Read the model definition and answer for the solid it produces. Units are mm, in the model's axes. Face numbers are marked on the shaded views. A direction names the side the tool comes from. Give positions to 0.01 mm unless a question says otherwise; leave off trailing zeros. Write each loop counter-clockwise with the first axis right and the second up, starting at its lowest first coordinate (ties: lowest second). Pieces come first, ordered by that corner, then holes. Notation, with made-up numbers: (3, -14.75) -> (35, -14.75) arc R8 cw to (35, -0.75) -> close; hole circle Ø4 at (66.25, 28.25). An arc over 180 degrees is marked (long way). Put each result on its own line as item: value. Start each with the question number.
Autodesk Inventor part; units mm, degrees
ref_plane "YZ Plane" through (0, 0, 0) normal (1, 0, 0) x (0, 1, 0)
ref_plane "XZ Plane" through (0, 0, 0) normal (0, 1, 0) x (-1, 0, 0)
ref_plane "XY Plane" through (0, 0, 0) normal (0, 0, 1) x (1, 0, 0)
sketch "Sketch1" plane through (0, 0, 0) normal (1, 0, 0) x (0, 1, 0)
  line L0 (0, 0) -> (20, 0)
  line L1 (20, 0) -> (20, -17)
  line L2 (20, -17) -> (0, -17)
  line L3 (0, -17) -> (0, 0)
  dimension "d0" = 20
  dimension "d1" = 17
extrude "Extrusion1" add sketch "Sketch1" along normal blind 3
sketch "Sketch2" plane through (0, 0, -17) normal (0, -1, 0) x (1, 0, 0)
  line L0 (3, 0) -> (3, 17)
  line L1 (3, 17) -> (-17, 17)
  line L2 (-17, 17) -> (-17, 0)
  line L3 (-17, 0) -> (3, 0)
  line L4 (3, 0) -> (3, 17)
  line L5 (-17, 17) -> (-17, 0)
  line L6 (0, 0) -> (-17, 0)
  line L7 (0, 17) -> (0, 0)
  line L8 (-17, 17) -> (0, 17)
  line L9 (-10, 8.5) -> (-7, 8.5) construction
  line L10 (-10, 5) -> (-7, 5)
  line L11 (-7, 12) -> (-10, 12)
  arc A0 (-10, 12) -> (-10, 5) centre (-10, 8.5) ccw
  arc A1 (-7, 5) -> (-7, 12) centre (-7, 8.5) ccw
  point P0 (0, 17)
  point P1 (0, 0)
  point P2 (-8.5, 8.5)
  dimension "d4" = 20
  dimension "d15" = 7
  dimension "d16" = 3
  dimension "d17" = 7
  dimension "d18" = 17
  dimension "d19" = 17
  dimension "d20" = 8.5
extrude "Extrusion2" add sketch "Sketch2" against normal blind 3 contours L3 L7 L1 L0 | L3 L2 L1 L7 | A0 L11 A1 L10
sketch "Sketch3" plane through (0, 0, 0) normal (-1, 0, 0) x (0, 0, 1)
  line L0 (-17, 3) -> (0, 3)
  line L1 (0, 20) -> (0, 3)
  line L2 (-17, 20) -> (0, 20)
  line L3 (-17, 3) -> (-17, 20)
  line L4 (-8.5, 10) -> (-8.5, 13) construction
  line L5 (-5, 10) -> (-5, 13)
  line L6 (-12, 13) -> (-12, 10)
  arc A0 (-12, 10) -> (-5, 10) centre (-8.5, 10) ccw
  arc A1 (-5, 13) -> (-12, 13) centre (-8.5, 13) ccw
  point P0 (0, 0)
  point P1 (-8.5, 11.5)
  dimension "d7" = 7
  dimension "d8" = 3
  dimension "d9" = 7
  dimension "d10" = 17
  dimension "d11" = 17
  dimension "d12" = 8.5
extrude "Extrusion3" cut sketch "Sketch3" against normal blind 3 contours A0 L6 A1 L5
extrude "Extrusion4" cut sketch "Sketch2" against normal blind 3 contours A0 L11 A1 L10
equation "\"d17\" = -0.5 * d16 + 0.5 * d18"
equation "\"d20\" = 0.5 * d19"
equation "\"d9\" = -0.5 * d8 + 0.5 * d10"
equation "\"d12\" = 0.5 * d11"
properties part number "2020RightAngle" material "Aluminum 6061"
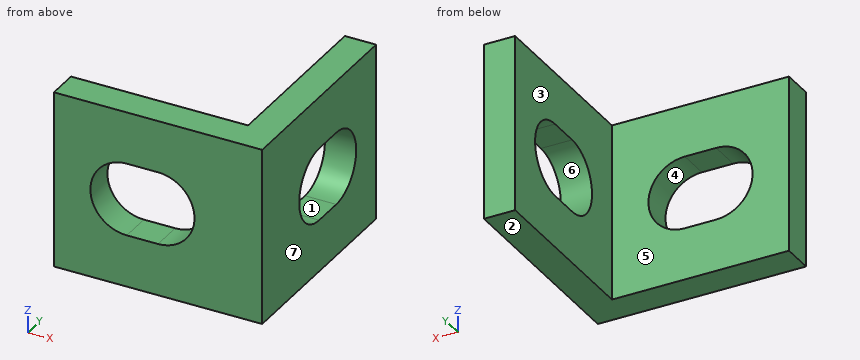
1) A cutting plane is placed at C-C on z = -4.5. Give the vertices of the cut face in (x, y).
2) For the marked faces 4, 5, 6 and 7, determine the directions among +Z, -Z, +X, -X, +Y, -Y from which every point of the face is accessible in a straight line to the end or side of a thin tool.
3) A cutting plane is placed at D-D on x = -15.5. Give the vertices of the cut face in (y, z).
4) For a pull along Z with two mould halves and no side action, classify the marked faces 1, 2 and 3 as pulls with the +Z half, pulls with the -Z half, needs draft (parallel to the pull), parting line crosses it, or undercut.
5) A cutting plane is placed at A-A on y = 12. Give the vertices of the cut face in (x, z).
6) Straight lines are drawn through the part: line 1 (X direction, y = 18, z = -3); line 2 (X direction, y = 2.75, z = -7.5). For each, find the intervals that lie inside material, in ascending order. Write a range as [from, to].
7) Each of these flat-tipped pins is pushed along its axis until it touches: pin 1 Ø12 at (x, y) = (-11, 12) entering from -Z; pin 2 Ø0.9 at (x, y) = (2, 11.5) entering from +Z; pin 3 Ø8.5 at (x, z) = (-5, -6.5) entering from +Y. Where does it stop, or does it pass through?
8) A cutting plane is placed at B-B on z = -6.75. Give the vertices of the cut face in (x, y).
Results found:
1. outline: (-17, 0) -> (3, 0) -> (3, 20) -> (0, 20) -> (0, 3) -> (-17, 3) -> close
2. face 4: +Y, -Y
2. face 5: +Z, -Z, -X, +Y
2. face 6: +X, -X
2. face 7: +Z, -Z, +X, +Y, -Y
3. outline: (0, -17) -> (3, -17) -> (3, 0) -> (0, 0) -> close
4. face 1: undercut
4. face 2: pulls with the -Z half
4. face 3: needs draft
5. outline: (0, -17) -> (3, -17) -> (3, -12) -> (0, -12) -> close; (0, -5) -> (3, -5) -> (3, 0) -> (0, 0) -> close
6. line 1: x = [0, 3]
6. line 2: x = [-17, -13.35], [-3.65, 3]
7. pin 1: passes through
7. pin 2: stops at z = 0
7. pin 3: stops at y = 3
8. outline: (-17, 0) -> (-13.03, 0) -> (-13.03, 3) -> (-17, 3) -> close; (-3.97, 0) -> (3, 0) -> (3, 6.97) -> (0, 6.97) -> (0, 3) -> (-3.97, 3) -> close; (0, 16.03) -> (3, 16.03) -> (3, 20) -> (0, 20) -> close
